```python
from build123d import *

# Parameters (mm, degrees)
ESTRUSIONE_ESTRUSIONE1_DEPTH = 180
SCHIZZO3_R                   = 17
TAGLIO_ESTRUSIONE2_DEPTH     = 183.295611683
SCHIZZO4_R                   = 15
ESTRUSIONE_ESTRUSIONE2_DEPTH = 25
ESTRUSIONE_ESTRUSIONE3_START = -2
SCHIZZO6_R                   = 15
ESTRUSIONE_ESTRUSIONE3_DEPTH = 2
TAGLIO_ESTRUSIONE4_REACH     = 211.92
TAGLIO_ESTRUSIONE5_REACH     = 211.843
ESTRUSIONE_ESTRUSIONE4_START = 1
SCHIZZO11_R                  = 15
ESTRUSIONE_ESTRUSIONE4_DEPTH = 1
SMUSSO1_SIZE                 = 2
SMUSSO1_SIZE_2               = 1.154700538
SMUSSO2_SIZE                 = 2
SCHIZZO12_R                  = 2.5
TAGLIO_ESTRUSIONE6_DEPTH     = 211.527047297
SCHIZZO13_R                  = 4.75
TAGLIO_ESTRUSIONE7_DEPTH     = 2
SCHIZZO14_R                  = 1.5
TAGLIO_ESTRUSIONE9_DEPTH     = 211.527047297
SCHIZZO15_R                  = 3.75
ESTRUSIONE_ESTRUSIONE5_DEPTH = 25
SCHIZZO16_R                  = 1.75
TAGLIO_ESTRUSIONE10_DEPTH    = 211.861655223
TAGLIO_ESTRUSIONE11_DEPTH    = 211.527047297


# Some blends are built 0.0001 mm under size
with BuildPart() as part:
    # Schizzo1 → Estrusione-Estrusione1 (new body)
    with BuildSketch(Plane.XY):
        Polygon((10.623281363, 5.122982669), (3.623281363, 15.122982669), (-7.376718637, 15.122982669), (-14.376718637, 5.122982669), (-14.376718637, 0.122982669), (-7.376718637, -9.877017331), (3.623281363, -9.877017331), (10.623281363, 0.122982669), align=None)
        Polygon((-12.376718637, 4.492538208), (-6.335407514, 13.122982669), (-2.876718637, 13.122982669), (-2.876718637, -7.877017331), (-6.335407514, -7.877017331), (-12.376718637, 0.753427131), align=None, mode=Mode.SUBTRACT)
        Polygon((2.58197024, -7.877017331), (-0.876718637, -7.877017331), (-0.876718637, 13.122982669), (2.58197024, 13.122982669), (8.623281363, 4.492538208), (8.623281363, 0.753427131), align=None, mode=Mode.SUBTRACT)
    extrude(amount=ESTRUSIONE_ESTRUSIONE1_DEPTH)

    # Schizzo3 → Taglio-Estrusione2 (cut, through all)
    with BuildSketch(Plane(origin=(0, 15.122982669, 0), x_dir=(1, 0, 0), z_dir=(0, 1, 0))):
        with Locations((-1.876718637, -191.521718622)):
            Circle(SCHIZZO3_R)
    extrude(amount=-TAGLIO_ESTRUSIONE2_DEPTH, mode=Mode.SUBTRACT)

    # Schizzo4 → Estrusione-Estrusione2 (add, through all)
    with BuildSketch(Plane(origin=(0, 15.122982669, 0), x_dir=(1, 0, 0), z_dir=(0, 1, 0))):
        with BuildLine():
            ThreePointArc((-7.376718637, -175.43601068), (-1.876718637, -208.521718622), (3.623281363, -175.43601068))
            ThreePointArc((3.623281363, -175.43601068), (-1.876718637, -174.521718622), (-7.376718637, -175.43601068))
        make_face()
        with Locations(Location((-1.876718637, -191.521718622, 0), (0, 0, 270))):
            Circle(SCHIZZO4_R, mode=Mode.SUBTRACT)
    extrude(amount=-ESTRUSIONE_ESTRUSIONE2_DEPTH)

    # Schizzo6 → Estrusione-Estrusione3 (add)
    with BuildSketch(Plane.XZ.offset(9.877017331).offset(ESTRUSIONE_ESTRUSIONE3_START)):
        with Locations(Location((-1.876718637, 191.521718622, 0), (0, 0, 90))):
            Circle(SCHIZZO6_R)
    extrude(amount=ESTRUSIONE_ESTRUSIONE3_DEPTH)

    # Schizzo8 → Taglio-Estrusione4 (cut, up to next)
    with BuildSketch(Plane(origin=(0, 0, 0), x_dir=(-1, 0, 0), z_dir=(0, 0, -1)), mode=Mode.PRIVATE) as taglio_estrusione4_sk1:
        Polygon((0.876718637, -7.877017331), (-2.58197024, -7.877017331), (-8.623281363, 0.753427131), (-8.623281363, 4.492538208), (-2.58197024, 13.122982669), (0.876718637, 13.122982669), align=None)
    taglio_estrusione4_tool1 = extrude(taglio_estrusione4_sk1.sketch, amount=-TAGLIO_ESTRUSIONE4_REACH, mode=Mode.PRIVATE) & part.part
    # Schizzo8 → Taglio-Estrusione4 (cut, up to next)
    with BuildSketch(Plane(origin=(0, 0, 0), x_dir=(-1, 0, 0), z_dir=(0, 0, -1)), mode=Mode.PRIVATE) as taglio_estrusione4_sk2:
        Polygon((2.876718637, -7.877017331), (2.876718637, 13.122982669), (6.335407514, 13.122982669), (12.376718637, 4.492538208), (12.376718637, 0.753427131), (6.335407514, -7.877017331), align=None)
    taglio_estrusione4_tool2 = extrude(taglio_estrusione4_sk2.sketch, amount=-TAGLIO_ESTRUSIONE4_REACH, mode=Mode.PRIVATE) & part.part
    add(taglio_estrusione4_tool1.solids().sort_by_distance((2.905149, 2.622983, 0))[0], mode=Mode.SUBTRACT)
    add(taglio_estrusione4_tool2.solids().sort_by_distance((-6.658586, 2.622983, 0))[0], mode=Mode.SUBTRACT)

    # Schizzo10 → Taglio-Estrusione5 (cut, up to next)
    with BuildSketch(Plane(origin=(-0.876718637, 0, 0), x_dir=(0, 0, -1), z_dir=(1, 0, 0)), mode=Mode.PRIVATE) as taglio_estrusione5_sk1:
        Polygon((-176.555089075, -7.877017331), (-176.555089075, 7.122982669), (-163.555089075, -7.877017331), align=None)
    taglio_estrusione5_tool1 = extrude(taglio_estrusione5_sk1.sketch, amount=-TAGLIO_ESTRUSIONE5_REACH, mode=Mode.PRIVATE) & part.part
    add(taglio_estrusione5_tool1.solids().sort_by_distance((-0.876719, -2.877017, 172.221756))[0], mode=Mode.SUBTRACT)

    # Schizzo11 → Estrusione-Estrusione4 (add)
    with BuildSketch(Plane(origin=(0, -7.877017331, 0), x_dir=(1, 0, 0), z_dir=(0, 1, 0)).offset(ESTRUSIONE_ESTRUSIONE4_START)):
        with Locations(Location((-1.876718637, -191.521718622, 0), (0, 0, 270))):
            Circle(SCHIZZO11_R)
    extrude(amount=-ESTRUSIONE_ESTRUSIONE4_DEPTH)

    # Smusso1
    # the kernel refuses this chamfer: 2, 1.154700538 mm, written as the material it adds along each edge
    with BuildSketch(Plane(origin=(-1.876718637, -7.877017331, 191.521718622), x_dir=(0.6026136012063945, 0, -0.7980331118700906), z_dir=(0.7980331118700906, 0, 0.6026136012063945))) as smusso1_piece_1_section:
        Polygon((15 + SMUSSO1_SIZE, 0), (15, SMUSSO1_SIZE_2), (15, 0), align=None)
    smusso1_piece_1 = revolve(axis=Axis((-1.876718637, -7.877017331, 191.521718622), (0, 1, 0)), revolution_arc=74.114626536, mode=Mode.PRIVATE)
    smusso1_piece_1 = split(smusso1_piece_1, bisect_by=Plane(origin=(5.278960516, -6.877017331, 177.600505235), z_dir=(0, -1, 0)), keep=Keep.TOP, mode=Mode.PRIVATE)
    add(smusso1_piece_1)

    # Smusso2
    smusso2_edges = [part.edges().sort_by_distance(p)[0] for p in [
        (-1.876718637, -9.877017331, 208.521718622),
    ]]
    chamfer(smusso2_edges, length=SMUSSO2_SIZE - 0.0001)  # a hair under: the kernel refuses the full size

    # Schizzo12 → Taglio-Estrusione6 (cut, through all)
    with BuildSketch(Plane(origin=(0, -6.877017331, 0), x_dir=(1, 0, 0), z_dir=(0, 1, 0))):
        with Locations(Location((-1.876718637, -191.521718622, 0), (0, 0, 270))):
            Circle(SCHIZZO12_R)
    extrude(amount=-TAGLIO_ESTRUSIONE6_DEPTH, mode=Mode.SUBTRACT)

    # Schizzo13 → Taglio-Estrusione7 (cut)
    with BuildSketch(Plane(origin=(0, -6.877017331, 0), x_dir=(1, 0, 0), z_dir=(0, 1, 0))):
        with Locations(Location((-1.876718637, -191.521718622, 0), (0, 0, 270))):
            Circle(SCHIZZO13_R)
    extrude(amount=-TAGLIO_ESTRUSIONE7_DEPTH, mode=Mode.SUBTRACT)

    # Schizzo14 → Taglio-Estrusione9 (cut, through all)
    with BuildSketch(Plane(origin=(0, -6.877017331, 0), x_dir=(1, 0, 0), z_dir=(0, 1, 0))):
        with Locations(Location((4.852993382, -198.227013257, 0), (0, 0, 270))):
            Circle(SCHIZZO14_R)
        with Locations(Location((-8.606430656, -184.816423987, 0), (0, 0, 270))):
            Circle(SCHIZZO14_R)
        with Locations(Location((-7.52328254, -197.188844533, 0), (0, 0, 270))):
            Circle(SCHIZZO14_R)
        with Locations(Location((3.769845266, -185.854592711, 0), (0, 0, 270))):
            Circle(SCHIZZO14_R)
    extrude(amount=-TAGLIO_ESTRUSIONE9_DEPTH, mode=Mode.SUBTRACT)

    # Schizzo15 → Estrusione-Estrusione5 (add)
    with BuildSketch(Plane(origin=(0, 15.122982669, 0), x_dir=(1, 0, 0), z_dir=(0, 1, 0))):
        with Locations((-1.876718637, -28)):
            Circle(SCHIZZO15_R)
        with Locations((-1.876718637, -9)):
            Circle(SCHIZZO15_R)
    extrude(amount=-ESTRUSIONE_ESTRUSIONE5_DEPTH)

    # Schizzo16 → Taglio-Estrusione10 (cut, through all)
    with BuildSketch(Plane(origin=(0, 15.122982669, 0), x_dir=(1, 0, 0), z_dir=(0, 1, 0))):
        with Locations(Location((-1.876718637, -28, 0), (0, 0, 270))):
            Circle(SCHIZZO16_R)
        with Locations(Location((-1.876718637, -9, 0), (0, 0, 270))):
            Circle(SCHIZZO16_R)
    extrude(amount=-TAGLIO_ESTRUSIONE10_DEPTH, mode=Mode.SUBTRACT)

    # Schizzo17 → Taglio-Estrusione11 (cut, through all)
    with BuildSketch(Plane(origin=(0, -6.877017331, 0), x_dir=(1, 0, 0), z_dir=(0, 1, 0))):
        with BuildLine():
            Line((-8.78535733, -190.040708293), (-13.650216694, -189.259165677))
            ThreePointArc((-13.650216694, -189.259165677), (-15.876718637, -191.521718622), (-13.650216694, -193.784271566))
            Line((-13.650216694, -193.784271566), (-8.78535733, -193.002728951))
            ThreePointArc((-8.78535733, -193.002728951), (-7.52328254, -191.521718622), (-8.78535733, -190.040708293))
        make_face()
        with BuildLine():
            Line((-0.395708308, -184.613079929), (0.385834308, -179.748220565))
            ThreePointArc((0.385834308, -179.748220565), (-1.876718637, -177.521718622), (-4.139271581, -179.748220565))
            Line((-4.139271581, -179.748220565), (-3.357728966, -184.613079929))
            ThreePointArc((-3.357728966, -184.613079929), (-1.876718637, -185.875154719), (-0.395708308, -184.613079929))
        make_face()
        with BuildLine():
            Line((5.031920056, -193.002728951), (9.89677942, -193.784271566))
            ThreePointArc((9.89677942, -193.784271566), (12.123281363, -191.521718622), (9.89677942, -189.259165677))
            Line((9.89677942, -189.259165677), (5.031920056, -190.040708293))
            ThreePointArc((5.031920056, -190.040708293), (3.769845266, -191.521718622), (5.031920056, -193.002728951))
        make_face()
        with BuildLine():
            Line((-3.357728966, -198.430357315), (-4.139271581, -203.295216678))
            ThreePointArc((-4.139271581, -203.295216678), (-1.876718637, -205.521718622), (0.385834308, -203.295216678))
            Line((0.385834308, -203.295216678), (-0.395708308, -198.430357315))
            ThreePointArc((-0.395708308, -198.430357315), (-1.876718637, -197.168282525), (-3.357728966, -198.430357315))
        make_face()
    extrude(amount=-TAGLIO_ESTRUSIONE11_DEPTH, mode=Mode.SUBTRACT)


solid = part.part
```
Work out the finished part from the listing and answer in its coordinate system (mm). A direction names the side the tool comes from. Give positions to 0.01 mm unless a question says otherwise; leave off trailing zeros. Order: outer loops, then holes, each group sorted by start corner. A loop starts at its lowest first (then second) coordinate and runs counter-clockwise, first axis right, second up. Notation, with made-up numbers: (84, 51) -> (89, 51) arc R14 ccw to (89, 56) -> close; hole circle Ø1 at (51.25, 42.25). An arc over 180 degrees is marked (long way). Answer as CSV lines item,"result". Start each with the question number.
(1) Section D-D, the plane y = -3.25 is taken. Write down the section's boundary in (x, z).
(2) Section B-B, the plane y = 10.5 is taken. Write down the section's boundary in (x, z).
(3) Each of these flat-tipped pins is pushed along its axis until it touches: pin 1 Ø4 at (x, y) = (-7, 0.5) entering from +Z; pin 2 Ø12 at (y, z) = (11.5, 49) entering from +X; pin 3 Ø10 at (x, z) = (-15, 169.5) entering from +Y. Where does it stop, or does it pass through?
(4) Section A-A, the plane z = 9 is taken. Write down the section's boundary in (x, y), plus the area to 3 significant figures.
(5) Section C-C, the plane z = 132 is taken. Write down the section's boundary in (x, y), plus the area to 3 significant figures.
(6) Consider line 1 along X through (y, z) = (4.5, 28); line 2 along Y through (x, z) = (-4, 129.5); line 3 along Z through (x, y) = (-2, 10.25). Determine where each line is inside the solid, lowest interval first.
(7) For a pull along Y with two mould halves and no side action, classify faces 5 (the flat face through (-2.877, 2, 3)), 6 (the flat face through (7.07, -4.95, 88.74)), 7 (the flat face through (-2, 3, 0)) as released by +Y, released by -Y, zero draft, split by the parting line, or undercut.
(8) Which of the six approach directions +Z, -Z, +X, -X, +Y, -Y give full straight-line access (tool end or side, diameter ignored) to faces 1 (the cylindrical face through (-3.7, -7.86, 195.91)), 2 (the flat face through (10.623, 3, 89)), 3 (the flat face through (5.645, 8.747, 89.139)), 4 (the flat face through (-2.877, 2, 18))?
Entries:
1,outline,"(-12.02, 0) -> (-9.57, 0) -> (-9.57, 178.65) arc R15 cw (long way) to (5.82, 178.65) -> (5.82, 0) -> (8.26, 0) -> (8.26, 177.88) arc R17 ccw (long way) to (-12.02, 177.88) -> close; (-2.88, 0) -> (-0.88, 0) -> (-0.88, 5.39) arc R3.75 ccw to (-0.88, 12.61) -> (-0.88, 24.39) arc R3.75 ccw to (-0.88, 31.61) -> (-0.88, 167.57) -> (-2.88, 167.57) -> (-2.88, 31.61) arc R3.75 ccw to (-2.88, 24.39) -> (-2.88, 12.61) arc R3.75 ccw to (-2.88, 5.39) -> close; hole circle Ø3.5 at (-1.88, 9); hole circle Ø3.5 at (-1.88, 28)"
2,outline,"(-10.61, 0) -> (-8.17, 0) -> (-8.17, 177.91) arc R15 cw (long way) to (4.42, 177.91) -> (4.42, 0) -> (6.86, 0) -> (6.86, 176.94) arc R17 ccw (long way) to (-10.61, 176.94) -> close; (-2.88, 0) -> (-0.88, 0) -> (-0.88, 5.39) arc R3.75 ccw to (-0.88, 12.61) -> (-0.88, 24.39) arc R3.75 ccw to (-0.88, 31.61) -> (-0.88, 176.56) arc R15 cw to (-2.88, 176.56) -> (-2.88, 31.61) arc R3.75 ccw to (-2.88, 24.39) -> (-2.88, 12.61) arc R3.75 ccw to (-2.88, 5.39) -> close; hole circle Ø3.5 at (-1.88, 9); hole circle Ø3.5 at (-1.88, 28)"
3,pin 1,"z = 208.23"
3,pin 2,"x = 10.36"
3,pin 3,"y = 11.38"
4,outline,"(-14.38, 0.12) -> (-7.38, -9.88) -> (-3.63, -9.88) -> (-3.63, 15.12) -> (-7.38, 15.12) -> (-14.38, 5.12) -> close; (-0.13, -9.88) -> (3.62, -9.88) -> (10.62, 0.12) -> (10.62, 5.12) -> (3.62, 15.12) -> (-0.13, 15.12) -> close; hole (-12.38, 0.75) -> (-6.34, -7.88) -> (-5.63, -7.88) -> (-5.63, 13.12) -> (-6.34, 13.12) -> (-12.38, 4.49) -> close; hole (1.87, -7.88) -> (2.58, -7.88) -> (8.62, 0.75) -> (8.62, 4.49) -> (2.58, 13.12) -> (1.87, 13.12) -> close"
4,area,"218 mm²"
5,outline,"(-14.38, 0.12) -> (-7.38, -9.88) -> (3.62, -9.88) -> (10.62, 0.12) -> (10.62, 5.12) -> (3.62, 15.12) -> (-7.38, 15.12) -> (-14.38, 5.12) -> close; hole (-12.38, 0.75) -> (-6.34, -7.88) -> (-2.88, -7.88) -> (-2.88, 13.12) -> (-6.34, 13.12) -> (-12.38, 4.49) -> close; hole (-0.88, -7.88) -> (2.58, -7.88) -> (8.62, 0.75) -> (8.62, 4.49) -> (2.58, 13.12) -> (-0.88, 13.12) -> close"
5,area,"190 mm²"
6,line 1,"-14.38 to -12.37, -5.63 to -3.63, -0.13 to 1.87, 8.62 to 10.62"
6,line 2,"-9.88 to -7.88, 13.12 to 15.12"
6,line 3,"0 to 7.25, 10.75 to 26.25, 29.75 to 176.52, 206.52 to 208.52"
7,face 5,"undercut"
7,face 6,"released by -Y"
7,face 7,"zero draft"
8,face 1,"+Y"
8,face 2,"-Z, +X, +Y, -Y"
8,face 3,"-Z"
8,face 4,"none"
